```python
from build123d import *

# Parameters (mm, degrees)
SKETCH3_R               = 35
SKETCH3_R_2             = 6.15
BOSS_EXTRUDE1_DEPTH     = 10
SKETCH4_R               = 17.5
SKETCH4_R_2             = 6.15
BOSS_EXTRUDE2_DEPTH     = 15
SKETCH5_R               = 6.15
BOSS_EXTRUDE3_DEPTH     = 3
SKETCH7_R               = 2.7
CUT_EXTRUDE1_DEPTH      = 6
CUT_EXTRUDE2_DEPTH      = 10
SKETCH9_R               = 1.65
CUT_EXTRUDE3_DEPTH      = 84.669466186
CUT_EXTRUDE3_DEPTH_BACK = 84.669466186
CUT_EXTRUDE4_DEPTH      = 8.75
CUT_EXTRUDE5_START      = 20
SKETCH11_R              = 2.8
CUT_EXTRUDE5_DEPTH      = 5
SKETCH17_R              = 2.1
CUT_EXTRUDE6_DEPTH      = 3.5
CUT_EXTRUDE7_DEPTH      = 4


with BuildPart() as part:
    # Sketch3 → Boss-Extrude1 (new body)
    with BuildSketch(Plane.XY):
        Circle(SKETCH3_R)
        Circle(SKETCH3_R_2, mode=Mode.SUBTRACT)
    extrude(amount=-BOSS_EXTRUDE1_DEPTH)

    # Sketch4 → Boss-Extrude2 (add)
    with BuildSketch(Plane(origin=(0, 0, -10), x_dir=(-1, 0, 0), z_dir=(0, 0, -1))):
        with Locations(Location((0, 0, 0), (0, 0, 180))):
            Circle(SKETCH4_R)
        with Locations(Location((0, 0, 0), (0, 0, 180))):
            Circle(SKETCH4_R_2, mode=Mode.SUBTRACT)
    extrude(amount=BOSS_EXTRUDE2_DEPTH)

    # Sketch5 → Boss-Extrude3 (add)
    with BuildSketch(Plane.XY):
        Circle(SKETCH5_R)
    extrude(amount=-BOSS_EXTRUDE3_DEPTH)

    # Sketch7 → Cut-Extrude1 (cut)
    with BuildSketch(Plane.XY):
        with Locations((-24.335313846, 14.05)):
            Circle(SKETCH7_R)
        with Locations((-24.335313846, -14.05)):
            Circle(SKETCH7_R)
        with Locations((0, -28.1)):
            Circle(SKETCH7_R)
        with Locations((24.335313846, -14.05)):
            Circle(SKETCH7_R)
        with Locations((24.335313846, 14.05)):
            Circle(SKETCH7_R)
        with Locations((0, 28.1)):
            Circle(SKETCH7_R)
    extrude(amount=-CUT_EXTRUDE1_DEPTH, mode=Mode.SUBTRACT)

    # Sketch8 → Cut-Extrude2 (cut)
    with BuildSketch(Plane.XY):
        with BuildLine():
            Line((-23.943567294, 25.528524933), (-34.08013476, 7.971475067))
            ThreePointArc((-34.08013476, 7.971475067), (-30.310889132, 17.5), (-23.943567294, 25.528524933))
        make_face()
        with BuildLine():
            Line((34.08013476, -7.971475067), (23.943567294, -25.528524933))
            ThreePointArc((23.943567294, -25.528524933), (30.310889132, -17.5), (34.08013476, -7.971475067))
        make_face()
    extrude(amount=-CUT_EXTRUDE2_DEPTH, mode=Mode.SUBTRACT)

    # Sketch9 → Cut-Extrude3 (cut, two sides)
    with BuildSketch(Plane(origin=(-29.011851027, 16.75, -10), x_dir=(0.8660254037844387, -0.4999999999999999, 0), z_dir=(0.49999999999999994, 0.8660254037844388, 0))) as cut_extrude3_sk:
        with Locations(Location((33.5, 7.5, 0), (0, 0, 180))):
            Circle(SKETCH9_R)
    extrude(amount=CUT_EXTRUDE3_DEPTH, mode=Mode.SUBTRACT)
    extrude(cut_extrude3_sk.sketch, amount=-CUT_EXTRUDE3_DEPTH_BACK, mode=Mode.SUBTRACT)

    # Sketch10 → Cut-Extrude4 (cut, symmetric)
    with BuildSketch(Plane(origin=(-29.011851027, 16.75, -10), x_dir=(0.8660254037844387, -0.4999999999999999, 0), z_dir=(0.49999999999999994, 0.8660254037844388, 0))):
        Polygon((35.174315781, 10.4), (31.825684219, 10.4), (30.151368439, 7.5), (31.825684219, 4.6), (35.174315781, 4.6), (36.848631561, 7.5), align=None)
    extrude(amount=CUT_EXTRUDE4_DEPTH, both=True, mode=Mode.SUBTRACT)

    # Sketch11 → Cut-Extrude5 (cut)
    with BuildSketch(Plane(origin=(-29.011851027, 16.75, -10), x_dir=(0.8660254037844387, -0.4999999999999999, 0), z_dir=(0.49999999999999994, 0.8660254037844388, 0)).offset(CUT_EXTRUDE5_START)):
        with Locations(Location((33.5, 7.5, 0), (0, 0, 180))):
            Circle(SKETCH11_R)
    cut_extrude5 = extrude(amount=-CUT_EXTRUDE5_DEPTH, mode=Mode.SUBTRACT)

    # Mirror1: Cut-Extrude5 across plane
    add(cut_extrude5.mirror(Plane(origin=(-29.011851027, 16.75, -10), x_dir=(0, 0, 1), z_dir=(0.49999999999999994, 0.8660254037844388, 0))), mode=Mode.SUBTRACT)

    # Sketch17 → Cut-Extrude6 (cut)
    with BuildSketch(Plane(origin=(0, 0, -10), x_dir=(-1, 0, 0), z_dir=(0, 0, -1))):
        with Locations((14.05, 24.335313846)):
            Circle(SKETCH17_R)
        with Locations((28.1, 0)):
            Circle(SKETCH17_R)
        with Locations(Location((-28.1, 0, 0), (0, 0, 180))):
            Circle(SKETCH17_R)
        with Locations(Location((-14.05, -24.335313846, 0), (0, 0, 180))):
            Circle(SKETCH17_R)
    extrude(amount=-CUT_EXTRUDE6_DEPTH, mode=Mode.SUBTRACT)

    # Sketch18 → Cut-Extrude7 (cut)
    with BuildSketch(Plane(origin=(0, 0, -10), x_dir=(-1, 0, 0), z_dir=(0, 0, -1))):
        Polygon((26.644714923, 18.05), (22.02591277, 18.05), (19.716511693, 14.05), (22.02591277, 10.05), (26.644714923, 10.05), (28.954116, 14.05), align=None)
        Polygon((-2.309401077, 32.1), (-4.618802154, 28.1), (-2.309401077, 24.1), (2.309401077, 24.1), (4.618802154, 28.1), (2.309401077, 32.1), align=None)
        Polygon((28.954116, -14.05), (26.644714923, -10.05), (22.02591277, -10.05), (19.716511693, -14.05), (22.02591277, -18.05), (26.644714923, -18.05), align=None)
        Polygon((2.309401077, -32.1), (4.618802154, -28.1), (2.309401077, -24.1), (-2.309401077, -24.1), (-4.618802154, -28.1), (-2.309401077, -32.1), align=None)
        Polygon((-26.644714923, -18.05), (-22.02591277, -18.05), (-19.716511693, -14.05), (-22.02591277, -10.05), (-26.644714923, -10.05), (-28.954116, -14.05), align=None)
        Polygon((-28.954116, 14.05), (-26.644714923, 10.05), (-22.02591277, 10.05), (-19.716511693, 14.05), (-22.02591277, 18.05), (-26.644714923, 18.05), align=None)
    extrude(amount=-CUT_EXTRUDE7_DEPTH, mode=Mode.SUBTRACT)


solid = part.part
```
Geometry: final body of the model. Coordinates: model frame, mm. A direction names the side the tool comes from. Round coordinates to 2 decimals unless told otherwise and drop trailing zeros. Write each loop counter-clockwise with the first axis right and the second up, starting at its lowest first coordinate (ties: lowest second). Pieces come first, ordered by that corner, then holes. Notation, with made-up numbers: M -25.5,26.5 L 29.5,26.5 A21 cw 29.5,57.5 Z; hole C 70,-34 d5. An arc over 180 degrees is marked long. Answer in a Markdown table with one row per item. Add a question column.
(1) Ray query, L1, parallel to Y at x = 0, z = -7.5; L2, parallel to Y at x = 0, z = -1.3; L3, parallel to Y at x = -28.1, z = -8.95. Return the intervals inside material, ascending.
(2) Cut plane A-A, the plane x = 14.05. Return the cut outline in (y, z), then the cut area to 3 significant figures.
(3) Reachability of faces 1 (the face through (-0.585, 25.464, -2.958)), 2 (the face through (-27.78, -16.08, -8.03)), 3 (the face through (-4, -6, -20.4)) from +Z, -Z, +X, -X, +Y, -Y: full face, straight path, thin tool, end or side. Return the list, or none.
(4) Cut plane B-B, the plane z = -12. Return the cut outline in (x, y).
(5) Cut plane D-D, the plane x = 28.1. Return the cut outline in (y, z).
(6) Cut plane C-C, the plane z = -7.5. Give the number of separate pieces and of enclosed holes in the cut face, then the cut area to 3 significant figures.
(7) Draft query along Z for faces 4 (the face through (15.019, -22.472, -8.274)), 5 (the face through (-28, 0, -6.5)), 6 (the face through (-1.48, -7.61, -18.93)). Return one class per face: pulls with the +Z half, pulls with the -Z half, needs draft (parallel to the pull), parting line crosses it, or undercut.
(8) Contact query for flat-ended pins moving along their axis: pin 1 (8 mm diameter, centred on x = 0, y = -27, fed in from -Z); pin 2 (4.5 mm diameter, centred on x = -25, z = -9, fed in from -Y); pin 3 (5.5 mm diameter, centred on x = 14.05, y = -24.34, fed in from +Z); pin 4 (4 mm diameter, centred on x = 0, y = -26.5, fed in from -Z). Output: stop coordinate, or through.
Established:
| question | item | result |
|---|---|---|
| 1 | L1 | -35 to -32.1, -24.1 to -6.15, 6.15 to 24.1, 32.1 to 35 |
| 1 | L2 | -35 to -30.8, -25.4 to 25.4, 30.8 to 35 |
| 1 | L3 | -20.87 to -15.53, -12.57 to -2.1, 2.1 to 12.57, 15.53 to 18.33 |
| 2 | outline | M -32.06,-10 L -26.44,-10 L -26.44,-6.5 L -22.24,-6.5 L -22.24,-10 L -10.43,-10 L -10.43,-25 L 10.43,-25 L 10.43,-10 L 32.06,-10 L 32.06,0 L -32.06,0 Z |
| 2 | area | 939 mm² |
| 3 | face 1 | +Z, -Z |
| 3 | face 2 | -Z |
| 3 | face 3 | none |
| 4 | outline | C 0,0 d35; hole C 0,0 d12.3 |
| 5 | outline | M -18.33,-10 L -15.53,-10 L -15.53,-6 L -12.57,-6 L -12.57,-10 L -2.1,-10 L -2.1,-6.5 L 2.1,-6.5 L 2.1,-10 L 12.57,-10 L 12.57,-6 L 15.53,-6 L 15.53,-10 L 20.87,-10 L 20.87,0 L -18.33,0 Z |
| 6 | separate pieces | 1 |
| 6 | enclosed holes | 11 |
| 6 | area | 3,300 mm² |
| 7 | face 4 | needs draft |
| 7 | face 5 | pulls with the -Z half |
| 7 | face 6 | undercut |
| 8 | pin 1 | z = -10 |
| 8 | pin 2 | y = -26.6 |
| 8 | pin 3 | z = 0 |
| 8 | pin 4 | z = -6 |
